Drawing for the job (mm, zero at the part's lowest x, y, z). A direction names the side the tool comes from. Round coordinates to 2 decimals unless told otherwise and drop trailing zeros. Loops run counter-clockwise (first coordinate to the right, second up) from the corner with the lowest first, then second, coordinate; pieces in that order, holes last. Notation, with made-up numbers: M 22.25,75.25 L 36.25,75.25 A23 cw 36.25,113.25 Z; hole C -6,50.25 d6. An arc over 180 degrees is marked long. Answer in a Markdown table with one row per item.
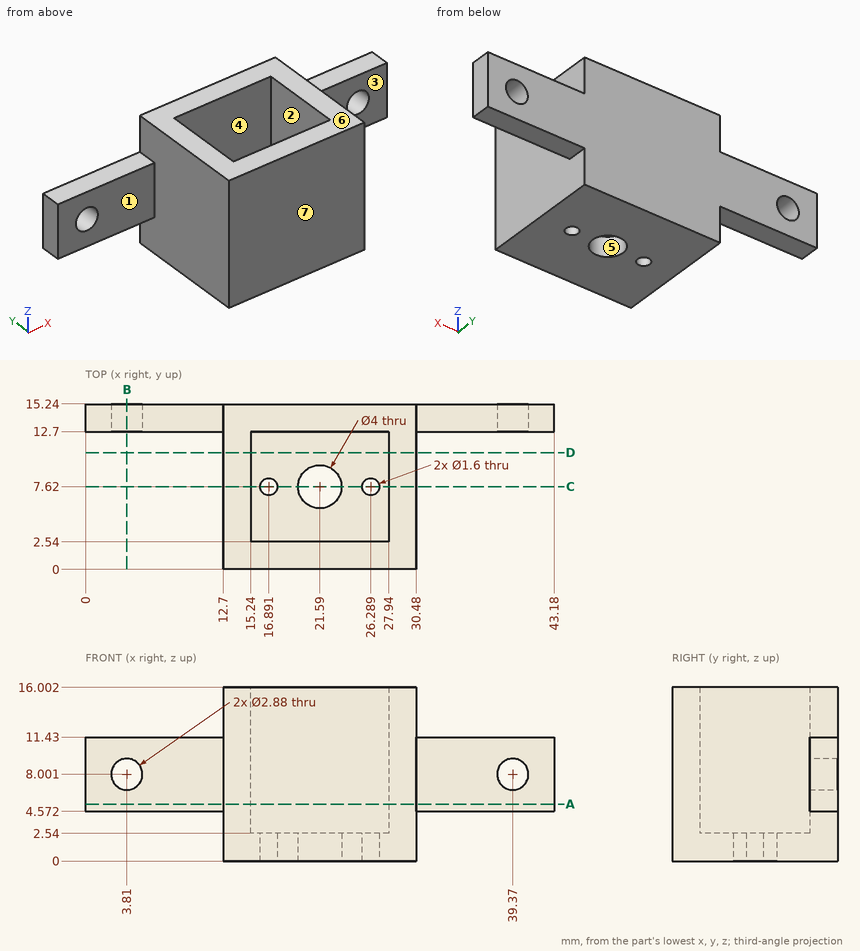
1. Saw through at B-B (x = 3.81). Write the cut outline in (y, z).
Verdict:
| item | result |
|---|---|
| outline | M 12.7,4.57 L 15.24,4.57 L 15.24,6.56 L 12.7,6.56 Z; M 12.7,9.44 L 15.24,9.44 L 15.24,11.43 L 12.7,11.43 Z |
2. Saw through at D-D (y = 10.75). Write the cut outline in (x, z), and give its area (3 significant figures).
Verdict:
| item | result |
|---|---|
| outline | M 12.7,0 L 30.48,0 L 30.48,16 L 27.94,16 L 27.94,2.54 L 15.24,2.54 L 15.24,16 L 12.7,16 Z |
| area | 114 mm² |
3. Pin check, flat tips, straight feed: pin 1 (1.5 mm diameter, centred on x = 37, z = 5.5, fed in from -Y); pin 2 (5 mm diameter, centred on y = 8.5, z = 12.5, fed in from -X); pin 3 (0.8 mm diameter, centred on x = 37.5, y = 14, fed in from +Z). Stop position of each tip, or through.
Verdict:
| item | result |
|---|---|
| pin 1 | stops at y = 12.7 |
| pin 2 | stops at x = 12.7 |
| pin 3 | stops at z = 11.43 |
4. Saw through at C-C (y = 7.62). Write the cut outline in (x, z).
Verdict:
| item | result |
|---|---|
| outline | M 12.7,0 L 16.09,0 L 16.09,2.54 L 15.24,2.54 L 15.24,16 L 12.7,16 Z; M 17.69,0 L 19.59,0 L 19.59,2.54 L 17.69,2.54 Z; M 23.59,0 L 25.49,0 L 25.49,2.54 L 23.59,2.54 Z; M 27.09,0 L 30.48,0 L 30.48,16 L 27.94,16 L 27.94,2.54 L 27.09,2.54 Z |
5. Wall check: probe 1 along X at (y, z) = (3.5, 3.5); probe 2 along Y at (x, z) = (18, 8.75); probe 3 along Y at (x, z) = (21.59, 0.5). Give the ranges that are in metal, low to high.
Verdict:
| item | result |
|---|---|
| probe 1 | x = 12.7 to 15.24, 27.94 to 30.48 |
| probe 2 | y = 0 to 2.54, 12.7 to 15.24 |
| probe 3 | y = 0 to 5.62, 9.62 to 15.24 |
6. Tool access for the marked faces 1, 2 and 3: list every direction of +Z, -Z, +X, -X, +Y, -Y with a clear straight run to the whole face (end or side of a thin tool).
Verdict:
| item | result |
|---|---|
| face 1 | +Z, -Z, -X, -Y |
| face 2 | +Z |
| face 3 | +Z, -Z, +X, -Y |
7. Saw through at A-A (z = 5.25). Write the cut outline in (x, y), and give its area (3 significant figures).
Verdict:
| item | result |
|---|---|
| outline | M 0,12.7 L 12.7,12.7 L 12.7,0 L 30.48,0 L 30.48,12.7 L 43.18,12.7 L 43.18,15.24 L 0,15.24 Z; hole M 15.24,2.54 L 27.94,2.54 L 27.94,12.7 L 15.24,12.7 Z |
| area | 206 mm² |
8. Mould opens along Y. For the marked faces 4, 5, 6 and 7 say: +Y half, -Y half, draft (parallel to the pull), parting line (faces both ways), or undercut.
Verdict:
| item | result |
|---|---|
| face 4 | undercut |
| face 5 | undercut |
| face 6 | draft |
| face 7 | -Y half |
